```python
from build123d import *

# Parameters (mm, degrees)
SKETCH_1_R      = 2
EXTRUDE_1_DEPTH = 0.75


with BuildPart() as part:
    # Эскиз1 → Бобышка-Вытянуть1 (new, symmetric)
    with BuildSketch(Plane.XY):
        with BuildLine():
            Line((-1.837638241, 9.854632004), (-1.837638241, 6.314293406))
            ThreePointArc((-1.837638241, 6.314293406), (-1.611630943, 5.178077993), (-0.968016612, 4.214841076))
            Line((-0.968016612, 4.214841076), (0.455254978, 2.791569486))
            ThreePointArc((0.455254978, 2.791569486), (1.162361759, 2.498676267), (1.869468541, 2.791569486))
            Line((1.869468541, 2.791569486), (3.292740131, 4.214841076))
            ThreePointArc((3.292740131, 4.214841076), (3.936354462, 5.178077993), (4.162361759, 6.314293406))
            Line((4.162361759, 6.314293406), (4.162361759, 9.854632004))
            ThreePointArc((4.162361759, 9.854632004), (3.936354462, 10.990847417), (3.292740131, 11.954084334))
            Line((3.292740131, 11.954084334), (1.869468541, 13.377355924))
            ThreePointArc((1.869468541, 13.377355924), (1.162361759, 13.670249143), (0.455254978, 13.377355924))
            Line((0.455254978, 13.377355924), (-0.968016612, 11.954084334))
            ThreePointArc((-0.968016612, 11.954084334), (-1.611630943, 10.990847417), (-1.837638241, 9.854632004))
        make_face()
        with Locations((1.162361759, 8.084462705)):
            Circle(SKETCH_1_R, mode=Mode.SUBTRACT)
    extrude(amount=EXTRUDE_1_DEPTH, both=True)


solid = part.part
```
Verification items for the finished model (mm, model axes). Give positions to 0.01 mm unless a question says otherwise; leave off trailing zeros. Order: outer loops, then holes, each group sorted by start corner. A loop starts at its lowest first (then second) coordinate and runs counter-clockwise, first axis right, second up. Notation, with made-up numbers: (-4.5, -4) -> (42.5, -4) arc R35 cw to (42.5, 31) -> close; hole circle Ø1 at (-35.5, 35.25). An arc over 180 degrees is marked (long way). One line per item, written item: value.
(1) Sectioned sample at B-B on z = 0.45. Record the cut outline in (x, y), then the cut area to 3 significant figures.
Final values:
outline: (-1.84, 6.31) arc R2.97 ccw to (-0.97, 4.21) -> (0.46, 2.79) arc R1 ccw to (1.87, 2.79) -> (3.29, 4.21) arc R2.97 ccw to (4.16, 6.31) -> (4.16, 9.85) arc R2.97 ccw to (3.29, 11.95) -> (1.87, 13.38) arc R1 ccw to (0.46, 13.38) -> (-0.97, 11.95) arc R2.97 ccw to (-1.84, 9.85) -> close; hole circle Ø4 at (1.16, 8.08)
area: 40.2 mm^2
(2) Sectioned sample at D-D on y = 3.5. Record the cut outline in (x, z), then the cut area to 3 significant figures.
Final values:
outline: (-0.25, -0.75) -> (2.58, -0.75) -> (2.58, 0.75) -> (-0.25, 0.75) -> close
area: 4.25 mm^2
(3) Gauge pin test, flat end, axial feed: pin 1 (3 mm diameter, centred on x = 1.16, y = 8.08, fed in from +Z). Record the tip position at first contact, or that the pin passes through.
Final values:
pin 1: through
(4) Sectioned sample at C-C on x = 2.25. Record the cut outline in (y, z).
Final values:
outline: (3.17, -0.75) -> (6.41, -0.75) -> (6.41, 0.75) -> (3.17, 0.75) -> close; (9.76, -0.75) -> (13, -0.75) -> (13, 0.75) -> (9.76, 0.75) -> close
(5) Sectioned sample at A-A on x = 1. Record the cut outline in (y, z).
Final values:
outline: (2.51, -0.75) -> (6.09, -0.75) -> (6.09, 0.75) -> (2.51, 0.75) -> close; (10.08, -0.75) -> (13.66, -0.75) -> (13.66, 0.75) -> (10.08, 0.75) -> close
(6) Draft check along X on faces 1 (the face through (-1.605, 11.006, 0.01)), 2 (the face through (0.73, 6.13, -0.01)), 3 (the face through (3.94, 10.98, 0.01)), 4 (the face through (-1, 8, 0.75)). Enter one of: pulls with the +X half, pulls with the -X half, needs draft (parallel to the pull), parting line crosses it, or undercut.
Final values:
face 1: pulls with the -X half
face 2: undercut
face 3: pulls with the +X half
face 4: needs draft
(7) Scan lines: line 1 along X through (y, z) = (8, 0.45); line 2 along Y through (x, z) = (0.25, 0.5); line 3 along Y through (x, z) = (2.75, -0.5). Record each from-to range of solid material in increasing order. Write a range as [from, to].
Final values:
line 1: [-1.84, -0.84], [3.16, 4.16]
line 2: [3, 6.3], [9.86, 13.17]
line 3: [3.67, 6.87], [9.3, 12.5]
